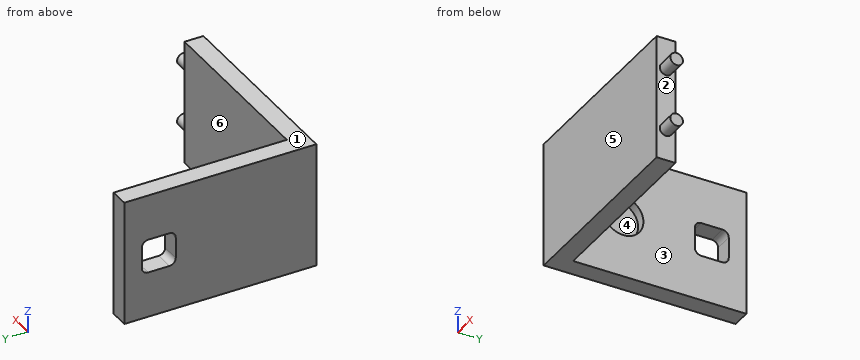
from build123d import *

# Parameters (mm, degrees)
Y_KSEKLIK_EKSTR_ZYON1_DEPTH = 100
IZIM4_R                     = 5
Y_KSEKLIK_EKSTR_ZYON2_DEPTH = 15
IZIM2_R                     = 16
KES_EKSTR_ZYON7_DEPTH       = 7.5
KES_EKSTR_ZYON8_DEPTH       = 16


with BuildPart() as part:
    # Çizim1 → Yükseklik-Ekstrüzyon1 (new body)
    with BuildSketch(Plane.XY):
        Polygon((-87.26990817, 0), (72.26990817, 0), (72.26990817, 15), (-72.26990817, 15), (-72.26990817, 153), (-87.26990817, 153), align=None)
    extrude(amount=-Y_KSEKLIK_EKSTR_ZYON1_DEPTH)

    # Çizim4 → Yükseklik-Ekstrüzyon2 (add)
    with BuildSketch(Plane(origin=(72.26990817, 0, 0), x_dir=(0, 0, -1), z_dir=(1, 0, 0))):
        with Locations((25, 7.5)):
            Circle(IZIM4_R)
        with Locations((75, 7.5)):
            Circle(IZIM4_R)
    extrude(amount=Y_KSEKLIK_EKSTR_ZYON2_DEPTH)

    # Çizim2 → Kes-Ekstrüzyon7 (cut)
    with BuildSketch(Plane(origin=(-72.26990817, 0, 0), x_dir=(0, 0, -1), z_dir=(1, 0, 0))):
        with Locations((50, 55)):
            Circle(IZIM2_R)
    extrude(amount=-KES_EKSTR_ZYON7_DEPTH, mode=Mode.SUBTRACT)

    # Çizim3 → Kes-Ekstrüzyon8 (cut, through all)
    with BuildSketch(Plane(origin=(-72.26990817, 0, 0), x_dir=(0, 0, -1), z_dir=(1, 0, 0))):
        with BuildLine():
            Line((41.5, 139), (58.5, 139))
            ThreePointArc((58.5, 139), (62.035533906, 137.535533906), (63.5, 134))
            Line((63.5, 134), (63.5, 117))
            ThreePointArc((63.5, 117), (62.035533906, 113.464466094), (58.5, 112))
            Line((58.5, 112), (41.5, 112))
            ThreePointArc((41.5, 112), (37.964466094, 113.464466094), (36.5, 117))
            Line((36.5, 117), (36.5, 134))
            ThreePointArc((36.5, 134), (37.964466094, 137.535533906), (41.5, 139))
        make_face()
    extrude(amount=-KES_EKSTR_ZYON8_DEPTH, mode=Mode.SUBTRACT)


solid = part.part
Verification items for the finished model (mm, model axes). Face numbers are marked on the shaded views. A direction names the side the tool comes from. Coordinates: 2 decimals unless noted, no trailing zeros. Loops run counter-clockwise (first coordinate to the right, second up) from the corner with the lowest first, then second, coordinate; pieces in that order, holes last. Notation, with made-up numbers: M -1.75,0 L 47.25,0 A23 ccw 47.25,35 Z; hole C 27.25,35.25 d6. An arc over 180 degrees is marked long. One line per item, written item: value.
1. Section check D-D on y = 78. Record the cut outline in (x, z), plus the area to 3 significant figures.
Answers follow:
outline: M -87.27,-100 L -72.27,-100 L -72.27,0 L -87.27,0 Z
area: 1,500 mm^2
2. Section check B-B on y = 55. Record the cut outline in (x, z).
Answers follow:
outline: M -87.27,-100 L -72.27,-100 L -72.27,-66 L -79.77,-66 L -79.77,-34 L -72.27,-34 L -72.27,0 L -87.27,0 Z
3. Set-up check for the marked faces 5 and 6: record each of +Z, -Z, +X, -X, +Y, -Y from which the full face is reachable in a straight line by a thin tool's end or side.
Answers follow:
face 5: +Z, -Z, +X, -X, -Y
face 6: +Z, -Z, +X, +Y
4. Section check C-C on x = -55.5. Record the cut outline in (y, z), plus the area to 3 significant figures.
Answers follow:
outline: M 0,-100 L 15,-100 L 15,0 L 0,0 Z
area: 1,500 mm^2
5. Section check A-A on z = -25. Record the cut outline in (x, y).
Answers follow:
outline: M -87.27,0 L 72.27,0 L 72.27,2.5 L 87.27,2.5 L 87.27,12.5 L 72.27,12.5 L 72.27,15 L -72.27,15 L -72.27,153 L -87.27,153 Z
6. Material ranges on line 1 along Y through (x, z) = (-75.5, -50); line 2 along X through (y, z) = (18, -52); line 3 along Y through (x, z) = (-15.5, -74), recorded low to high. Write a range as from..to.
Answers follow:
line 1: 0..39, 71..112, 139..153
line 2: -87.27..-72.27
line 3: 0..15
7. Mould release check, pull along Z, two halves, no side actions. Record for the marked faces 1, 2, 3 and 4: pulls with the +Z half, pulls with the -Z half, needs draft (parallel to the pull), parting line crosses it, or undercut.
Answers follow:
face 1: pulls with the +Z half
face 2: undercut
face 3: needs draft
face 4: undercut
8. Gauge pin test, flat ends, axial feed: P1, Ø12, axis at x = -31.5, z = -82, coming from the +Y side; P2, Ø12, axis at x = -37.5, y = 26, coming from the +Z side; P3, Ø7.5, axis at x = -81.5, z = -48, coming from the -Y side; P4, Ø16.5, axis at y = 7.5, z = -46, coming from the +X side. Record the tip position at first contact, or that the pin passes through.
Answers follow:
P1: y = 15
P2: through
P3: y = 0
P4: x = 72.27
